The figure shows three views and two pictorial views of one solid part (mm, origin at its lowest corner). Answer the questions. Coordinates: 2 decimals unless noted, no trailing zeros. Write each loop counter-clockwise with the first axis right and the second up, starting at its lowest first coordinate (ties: lowest second). Pieces come first, ordered by that corner, then holes.
Item 1: Each of these flat-tipped pins is pushed along its axis until it touches: P1, Ø1, axis at x = 32.5, y = 1.5, coming from the -Z side; P2, Ø1, axis at x = 32.5, y = 2, coming from the +Z side. Where does it stop, or does it pass through?
Item 2: Section B-B (x = 31.75) is taken. Give the vertices of the cut face in (y, z) (1 decimal), then the cut area to 3 significant figures.
Item 3: Section A-A (y = 2.65) is taken. Give the vertices of the cut face in (x, z).
Item 4: Straight lines are drawn through the part: probe 1 along X at (y, z) = (1.25, 77); probe 2 along Z at (x, y) = (43, 2.3) (1 decimal); probe 3 along Z at (x, y) = (13, 1.75) (1 decimal). For each, find the intervals that lie inside material, in ascending order.
Item 5: Section C-C (z = 65) is taken. Give the vertices of the cut face in (x, y) (1 decimal), then the cut area to 3 significant figures.
Item 6: Section D-D (x = 58.5) is taken. Give the vertices of the cut face in (y, z) (1 decimal).
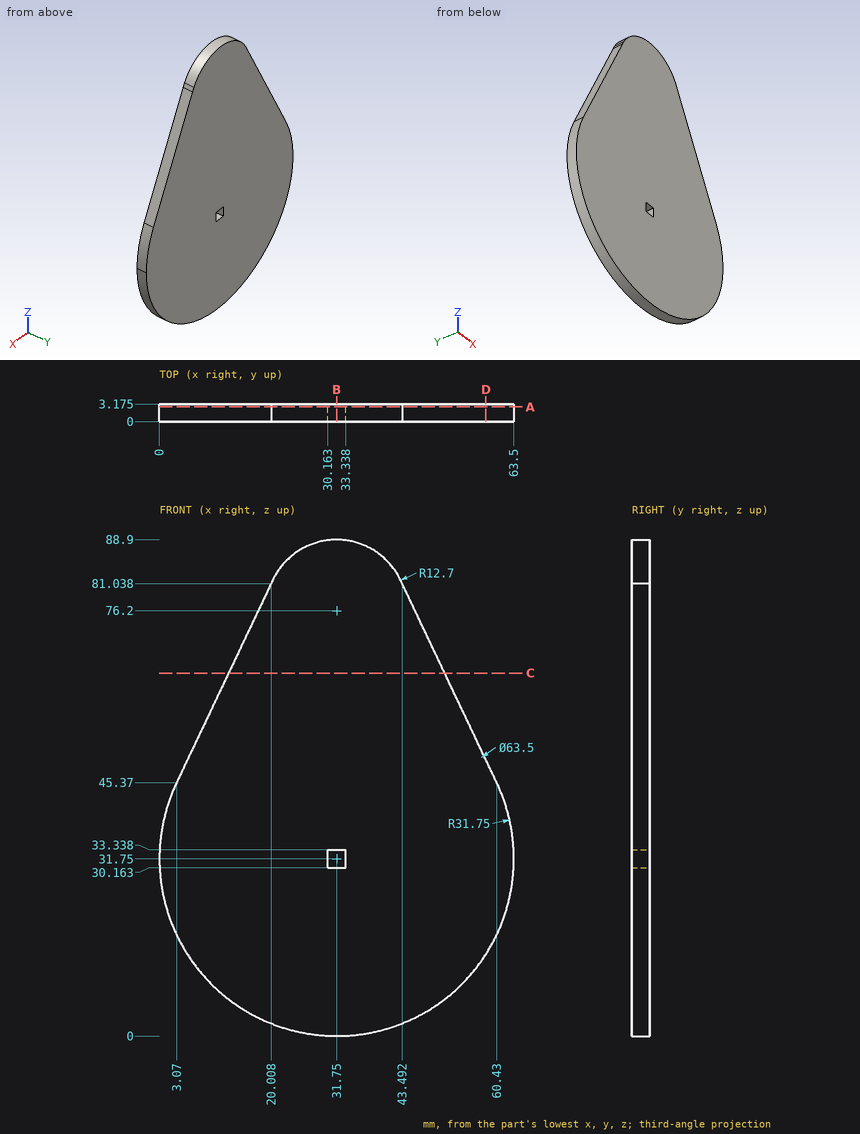
Established:
1. P1: stops at z = 0
1. P2: stops at z = 88.9
2. outline: (0, 0) - (3.2, 0) - (3.2, 30.2) - (0, 30.2) - close; (0, 33.3) - (3.2, 33.3) - (3.2, 88.9) - (0, 88.9) - close
2. area: 272 mm2
3. outline: (3.07, 45.37) arc R31.75 ccw (long way) to (60.43, 45.37) - (43.49, 81.04) arc R12.7 ccw to (20.01, 81.04) - close; hole (30.16, 30.16) - (33.34, 30.16) - (33.34, 33.34) - (30.16, 33.34) - close
4. probe 1: x = 18.09 to 45.41
4. probe 2: z = 2.1 to 82.1
4. probe 3: z = 6.1 to 66.3
5. outline: (12.4, 0) - (51.1, 0) - (51.1, 3.2) - (12.4, 3.2) - close
5. area: 123 mm2
6. outline: (0, 14.6) - (3.2, 14.6) - (3.2, 49.4) - (0, 49.4) - close
